Geometry: final body of the model. Coordinates: model frame, mm. Face numbers are marked on the shaded views. Give positions to 0.01 mm unless a question says otherwise; leave off trailing zeros. Write each loop counter-clockwise with the first axis right and the second up, starting at its lowest first coordinate (ties: lowest second). Pieces come first, ordered by that corner, then holes.
Q1. Pin query (flat end, axial travel): pin 1 Ø1 at (x, y) = (1, 2) entering from -Z; pin 2 Ø0.6 at (x, z) = (0.5, -0.5) entering from -Y; pin 3 Ø1 at (x, z) = (1, 0) entering from +Y. Return the tip coordinate at first contact, or that it passes through.
Q2. Mould query, pull axis Z, two halves, no side actions, for the marked faces 1, 2 and 3. Classes: +Z half, -Z half, draft (parallel to the pull), parting line (faces both ways), or undercut.
Q3. Section A-A (x = 1.15). Return the cut outline in (y, z).
Q4. Section C-C (y = 2). Return the cut outline in (x, z), plus the area to 3 significant figures.
Q5. Section B-B (z = -15.5). Return the cut outline in (x, y), plus the area to 3 significant figures.
Q6. Section D-D (z = -2.5). Return the cut outline in (x, y).
Q7. Line query: line 1 (Z direction, x = 1.75, y = -4.25); line 2 (Y direction, x = 0.1, z = 0); line 3 (Y direction, x = 1.6, z = -7). Output: solid intervals per line, ascending.
from build123d import *

# Parameters (mm, degrees)
SKETCH1_R           = 2
BOSS_EXTRUDE1_DEPTH = 2


with BuildPart() as part:
    # Sketch1 → Boss-Extrude1 (new body)
    with BuildSketch(Plane(origin=(0, 0, 0), x_dir=(0, 0, -1), z_dir=(1, 0, 0))):
        with BuildLine():
            Line((1, -5), (1, -3))
            Line((1, -3), (-1, -3))
            Line((-1, -3), (-1, 3))
            Line((-1, 3), (1, 3))
            Line((1, 3), (1, 5))
            Line((1, 5), (16, -1))
            ThreePointArc((16, -1), (20.196407848, -5.50210357), (15, -8.8))
            Line((15, -8.8), (1, -5))
        make_face()
        with Locations((16.228881189, -4.993446306)):
            Circle(SKETCH1_R, mode=Mode.SUBTRACT)
    extrude(amount=BOSS_EXTRUDE1_DEPTH)


solid = part.part
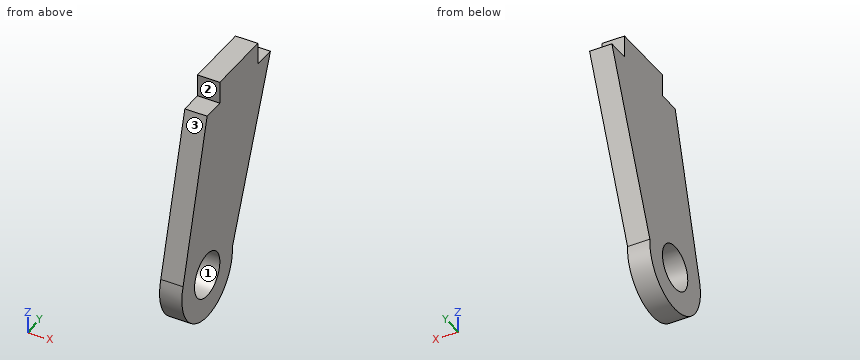
Computed:
1. pin 1: stops at z = -9.75
1. pin 2: stops at y = -3
1. pin 3: stops at y = 3
2. face 1: undercut
2. face 2: draft
2. face 3: +Z half
3. outline: (-8.8, -15) arc R4 ccw (long way) to (-1, -16) - (5, -1) - (3, -1) - (3, 1) - (-3, 1) - (-3, -1) - (-5, -1) - close; hole circle Ø4 at (-4.99, -16.23)
4. outline: (0, -8.5) - (2, -8.5) - (2, 1) - (0, 1) - close
4. area: 19.0 mm2
5. outline: (0, -8.93) - (2, -8.93) - (2, -6.86) - (0, -6.86) - close; (0, -3.13) - (2, -3.13) - (2, -0.8) - (0, -0.8) - close
5. area: 8.80 mm2
6. outline: (0, -5.41) - (2, -5.41) - (2, 4.4) - (0, 4.4) - close
7. line 1: z = -20.16 to -18.09, -14.37 to -1
7. line 2: y = -3 to 3
7. line 3: y = -6.63 to 2.6
